For this review, take the finished solid that the model builds, in its own axes (mm). A direction names the side the tool comes from. Give positions to 0.01 mm unless a question says otherwise; leave off trailing zeros. Loops run counter-clockwise (first coordinate to the right, second up) from the corner with the lowest first, then second, coordinate; pieces in that order, holes last. Notation, with made-up numbers: (-13, 18.5) - (13, 18.5) arc R22 cw to (13, 25.5) - close; hole circle Ø3 at (38.25, 59). An arc over 180 degrees is marked (long way). Use CSV: the item, a comma, the result in double quotes. Start each with the question number.
1. Take a section at B-B on x = -24.5. Give the boundary of the cut face in (y, z).
2. Wall thickness on line 1 (Y direction, x = 50.5, z = 47); line 2 (Y direction, x = -24.5, z = 64); line 3 (X direction, y = 16.5, z = 20): over which ranges is each line inside the solid? List them lowest first.
3. Take a section at A-A on y = 38. Give the boundary of the cut face in (x, z).
4. For pin 1 (4 mm diameter, centred on x = 40, y = 48, fed in from +Z); pin 2 (9 mm diameter, centred on x = 34.5, z = 43, fed in from -Y); pin 3 (2.5 mm diameter, centred on y = 114.5, z = 92, fed in from +X), all flat-tipped, find the tip position at first contact; note any pin that passes through.
5. Mouldability with a two-part tool opening along Y and no side actions: class faces 1 (the flat face through (9, 70, 94)), 2 (the flat face through (15.1, 168, 24.9)), 3 (the flat face through (-37.5, 117, 94)) as pulls with the +Y half, pulls with the -Y half, needs draft (parallel to the pull), parting line crosses it, or undercut.
6. Take a section at D-D on z = 19. Give the boundary of the cut face in (x, y).
7. For faces 4 (the flat face through (57.5, 117, 94)), 5 (the flat face through (-19, 20, 38)), 6 (the cylindrical face through (-24.891, 168.451, 47.974)), 7 (the flat face through (-39, 43, 13)), list the 3-axis set-ups (+Z, -Z, +X, -X, +Y, -Y) from which the entire face can be reached by the end or side of a thin tool; tool diameter is ignored.
8. Take a section at C-C on y = 116.5. Give the boundary of the cut face in (x, z), plus the area to 3 significant figures.
Autodesk Inventor part; units mm, degrees
ref_plane "Work Plane1" through (-48, 65, 2) normal (0, -1, 0) x (1, 0, 0)
ref_plane "Work Plane3" through (-48, 165, 5) normal (0, 1, 0) x (1, 0, 0)
ref_plane "Work Plane2" through (-48, 165, 5) normal (0, 1, 0) x (1, 0, 0)
sketch "Sketch2" plane through (0, 0, 0) normal (0, 0, 1) x (1, 0, 0)
  line L0 (0, 0) -> (70, 0)
  line L1 (70, 0) -> (70, 165)
  line L2 (70, 165) -> (0, 165)
  line L3 (0, 165) -> (0, 0)
  dimension "d0" = 165
  dimension "d1" = 70
extrude "Extrusion1" add sketch "Sketch2" along normal blind 90
sketch "Sketch6" plane through (0, 0, 0) normal (-1, 0, 0) x (0, 0, 1)
  line L0 (90, 0) -> (90, 165)
  line L1 (0, 0) -> (0, 165)
  line L2 (90, 165) -> (0, 165)
  line L3 (0, 165) -> (0, 65)
  line L4 (0, 65) -> (90, 65)
  line L5 (90, 65) -> (90, 165)
  dimension "d8" = 100
extrude "Extrusion3" add sketch "Sketch6" along normal blind 50
sketch "Sketch7" plane through (0, 65, 0) normal (0, -1, 0) x (1, 0, 0)
  line L0 (70, 90) -> (-50, 90)
  line L1 (0, 0) -> (0, 90)
  line L2 (-50, 90) -> (0, 90)
  line L3 (0, 90) -> (0, 38)
  line L4 (0, 38) -> (-50, 38)
  line L5 (-50, 38) -> (-50, 90)
  dimension "d11" = 52
extrude "Extrusion4" add sketch "Sketch7" along normal blind 75
sketch "Sketch8" plane through (0, 65, 38) normal (0, 0, -1) x (-1, 0, 0)
  line L0 (0, 0) -> (50, 0)
  line L1 (50, 0) -> (29, 0)
  line L2 (29, 0) -> (29, -45)
  line L3 (29, -45) -> (50, -45)
  line L4 (50, -45) -> (50, 0)
  point P0 (0, -65)
  point P1 (29, 0)
  dimension "d14" = 21
  dimension "d15" = 45
extrude "Extrusion5" add sketch "Sketch8" along normal blind 25
sketch "Sketch9" plane through (0, 0, 90) normal (0, 0, 1) x (1, 0, 0)
  line L0 (70, 165) -> (-50, 165)
  line L1 (-50, 165) -> (70, 165)
  line L2 (70, 165) -> (10, 165)
  line L3 (10, 70) -> (57.5, 70)
  line L4 (57.5, 70) -> (-37.5, 70)
  line L5 (-37.5, 70) -> (-37.5, 165)
  line L6 (57.5, 70) -> (57.5, 165)
  point P0 (0, 0)
  dimension "d20" = 95
  dimension "d21" = 95
extrude "Extrusion6" add sketch "Sketch9" along normal blind 8
ref_plane "Work Plane1" through (-48, 65, 2) normal (0, -1, 0) x (1, 0, 0)
sketch "Sketch10" plane through (-48, 65, 2) normal (0, -1, 0) x (1, 0, 0)
  line L0 (21, 34) -> (46, 34)
  line L1 (33.5, 34) -> (33.5, 0)
  line L2 (46, 0) -> (0, 0)
  circle A0 centre (33.5, 17) radius 12.5
  point P0 (48, -2)
extrude "Extrusion7" add sketch "Sketch10" along normal blind 70
ref_plane "Work Plane3" through (-48, 165, 5) normal (0, 1, 0) x (1, 0, 0)
sketch "Sketch11" plane through (-48, 165, 5) normal (0, 1, 0) x (1, 0, 0)
  line L0 (113, 0) -> (113, -80)
  line L1 (0, -80) -> (0, 0)
  circle A0 centre (56.5, -40) radius 21
  point P0 (48, 5)
  dimension "d29" = 42
extrude "Extrusion8" add sketch "Sketch11" along normal blind 6
ref_plane "Work Plane2" through (-48, 165, 5) normal (0, 1, 0) x (1, 0, 0)
sketch "Sketch12" plane through (-48, 165, 5) normal (0, 1, 0) x (1, 0, 0)
  circle A0 centre (56.5, -40) radius 21
  line L0 (35.5, -40) -> (26.5, -40)
  circle A1 centre (23.5, -40) radius 3
  point P0 (48, 5)
  dimension "d32" = 9
extrude "Extrusion9" add sketch "Sketch12" along normal blind 7 contours A1
sketch "Sketch13" plane through (8.5, 171, 45) normal (0, 1, 0) x (1, 0, 0)
  circle A0 centre (0, 0) radius 22.5
  arc A1 (21.4111, -6.9148) -> (21.4111, 6.9148) centre (22.5, 0) ccw
  point P0 (-8.5, 45)
  dimension "d37" = 45
  dimension "d38" = 14
extrude "Extrusion10" add sketch "Sketch13" along normal mid plane 6 contours A0
extrude "Extrusion11" add sketch "Sketch13" along normal blind 2 contours A0 A1
properties part number "windshield washer"
Check result:
1,outline,"(-10, 38) - (65, 38) - (65, 26.5) - (-5, 26.5) - (-5, 11.5) - (65, 11.5) - (65, 0) - (165, 0) - (165, 42) - (172, 42) - (172, 48) - (165, 48) - (165, 98) - (70, 98) - (70, 90) - (-10, 90) - close"
2,line 1,"y = 0 to 165"
2,line 2,"y = -10 to 165"
2,line 3,"x = -26.96 to -2.04, 0 to 70"
3,outline,"(-50, 13) - (-29, 13) - (-29, 38) - (0, 38) - (0, 0) - (70, 0) - (70, 90) - (-50, 90) - close; circle Ø25 at (-14.5, 19)"
4,pin 1,"stops at z = 90"
4,pin 2,"stops at y = 0"
4,pin 3,"stops at x = 57.5"
5,face 1,"pulls with the -Y half"
5,face 2,"undercut"
5,face 3,"needs draft"
6,outline,"(-50, 20) - (-29, 20) - (-29, 65) - (-27, 65) - (-27, -5) - (-2, -5) - (-2, 65) - (0, 65) - (0, 0) - (70, 0) - (70, 165) - (-50, 165) - close"
7,face 4,"+Z, +X, +Y, -Y"
7,face 5,"-Y"
7,face 6,"+Y"
7,face 7,"-Z, -X, -Y"
8,outline,"(-50, 0) - (70, 0) - (70, 90) - (57.5, 90) - (57.5, 98) - (-37.5, 98) - (-37.5, 90) - (-50, 90) - close"
8,area,"11,600 mm²"
